Read the model definition and answer for the solid it produces. Units are mm, in the model's axes. Coordinates: 2 decimals unless noted, no trailing zeros. Loops run counter-clockwise (first coordinate to the right, second up) from the corner with the lowest first, then second, coordinate; pieces in that order, holes last. Notation, with made-up numbers: M -14.75,1.5 L 31.25,1.5 A30 cw 31.25,31.5 Z; hole C 62.25,81 d10. An arc over 180 degrees is marked long. Put each result on its own line as item: value.
Autodesk Inventor part; units mm, degrees
ref_plane "YZ Plane" through (0, 0, 0) normal (1, 0, 0) x (0, 1, 0)
ref_plane "XZ Plane" through (0, 0, 0) normal (0, 1, 0) x (-1, 0, 0)
ref_plane "XY Plane" through (0, 0, 0) normal (0, 0, 1) x (1, 0, 0)
sketch "Esquisse1" plane through (0, 0, 0) normal (0, 1, 0) x (-1, 0, 0)
  line L0 (350, 500) -> (-350, 500)
  line L1 (-350, 500) -> (-350, -500)
  line L2 (-350, -500) -> (350, -500)
  line L3 (350, -500) -> (350, 500)
  point P0 (0, 0)
  dimension "d0" = 1000
  dimension "d1" = 700
  dimension "d2" = 350
  dimension "d3" = 500
extrude "Extrusion1" add sketch "Esquisse1" along normal blind 10
sketch "Esquisse2" plane through (0, 10, 0) normal (0, 1, 0) x (1, 0, 0)
  point P0 (0, 0)
sketch "Esquisse3" plane through (0, 10, 0) normal (0, 1, 0) x (1, 0, 0)
  point P0 (0, 0)
sketch "Esquisse4" plane through (0, 10, 0) normal (0, 1, 0) x (1, 0, 0)
  circle A0 centre (200, -380) radius 27.5
  line L0 (-350, -500) -> (350, -500)
  line L1 (350, -500) -> (350, 500)
  point P0 (0, 0)
  dimension "d6" = 55
  dimension "d7" = 120
  dimension "d8" = 150
extrude "Extrusion2" cut sketch "Esquisse4" against normal through all
sketch "Esquisse5" plane through (0, 10, 0) normal (0, 1, 0) x (1, 0, 0)
  circle A0 centre (-325, -475) radius 1.5
  circle A1 centre (325, -475) radius 1.5
  circle A2 centre (325, 475) radius 1.5
  circle A3 centre (-325, 475) radius 1.5
  line L0 (350, 500) -> (-350, 500)
  line L1 (350, -500) -> (350, 500)
  line L2 (-350, 500) -> (-350, -500)
  line L3 (-350, -500) -> (350, -500)
  circle A4 centre (-345, -190) radius 1.5
  circle A5 centre (-345, 190) radius 1.5
  circle A6 centre (0, -495) radius 1.5
  circle A7 centre (0, 495) radius 1.5
  circle A8 centre (345, -190) radius 1.5
  circle A9 centre (345, 190) radius 1.5
  point P0 (0, 0)
  dimension "d11" = 3
  dimension "d12" = 3
  dimension "d13" = 3
  dimension "d14" = 3
  dimension "d15" = 25
  dimension "d16" = 25
  dimension "d17" = 25
  dimension "d18" = 25
  dimension "d19" = 25
  dimension "d20" = 25
  dimension "d21" = 25
  dimension "d22" = 25
  dimension "d23" = 3
  dimension "d24" = 3
  dimension "d25" = 3
  dimension "d26" = 3
  dimension "d27" = 3
  dimension "d28" = 3
  dimension "d29" = 5
  dimension "d30" = 5
  dimension "d31" = 5
  dimension "d32" = 5
  dimension "d33" = 5
  dimension "d34" = 5
  dimension "d35" = 350
  dimension "d36" = 350
  dimension "d37" = 190
  dimension "d38" = 190
  dimension "d39" = 190
  dimension "d40" = 190
extrude "Extrusion3" cut sketch "Esquisse5" against normal through all contours A0 | A1 | A2 | A3 | A4 | A5 | A6 | A7 | A8 | A9
equation "\"d0\" = Longueur_Plateau"
equation "\"d1\" = Largeur_Plateau"
equation "\"d12\" = d11"
equation "\"d13\" = d11"
equation "\"d14\" = d11"
equation "\"d16\" = d15"
equation "\"d17\" = d15"
equation "\"d18\" = d15"
equation "\"d19\" = d15"
equation "\"d20\" = d15"
equation "\"d21\" = d15"
equation "\"d22\" = d15"
equation "\"d24\" = d23"
equation "\"d25\" = d23"
equation "\"d26\" = d23"
equation "\"d27\" = d23"
equation "\"d28\" = d23"
equation "\"d30\" = d29"
equation "\"d31\" = d29"
equation "\"d32\" = d29"
equation "\"d33\" = d29"
equation "\"d34\" = d29"
equation "\"Longueur_Plateau\" = 1000"
equation "\"Largeur_Plateau\" = 700"
properties part number "Plateau" material "Bois (bouleau)"
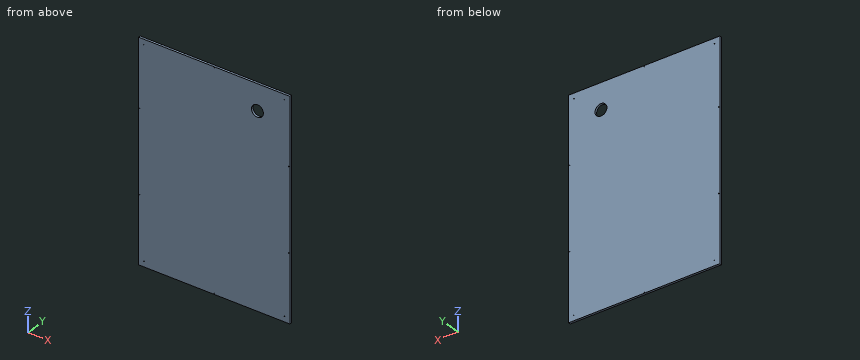
1) Straight lines are drawn through the part: line 1 (X direction, y = 7.5, z = 190); line 2 (Z direction, x = -325, y = 5); line 3 (X direction, y = 5.5, z = -495). For each, find the intervals that lie inside material, in ascending order. Write a range as [from, to].
Answer list:
line 1: x = [-350, -346.5], [-343.5, 343.5], [346.5, 350]
line 2: z = [-500, -476.5], [-473.5, 473.5], [476.5, 500]
line 3: x = [-350, -1.5], [1.5, 350]
2) Find section B-B, the plane z = 380. Write down the section's boundary in (x, y), plus the area to 3 significant figures.
Answer list:
outline: M -350,0 L 172.5,0 L 172.5,10 L -350,10 Z; M 227.5,0 L 350,0 L 350,10 L 227.5,10 Z
area: 6,450 mm^2
3) Given pin 1 Ø1.8 at (x, z) = (-345, -190) entering from -Y, flat-ended and moving along its own axis, determine where the tip first touches the part or whether it passes through.
Answer list:
pin 1: passes through
4) Find section A-A, the plane x = 200. Write down the section's boundary in (y, z).
Answer list:
outline: M 0,-500 L 10,-500 L 10,352.5 L 0,352.5 Z; M 0,407.5 L 10,407.5 L 10,500 L 0,500 Z
